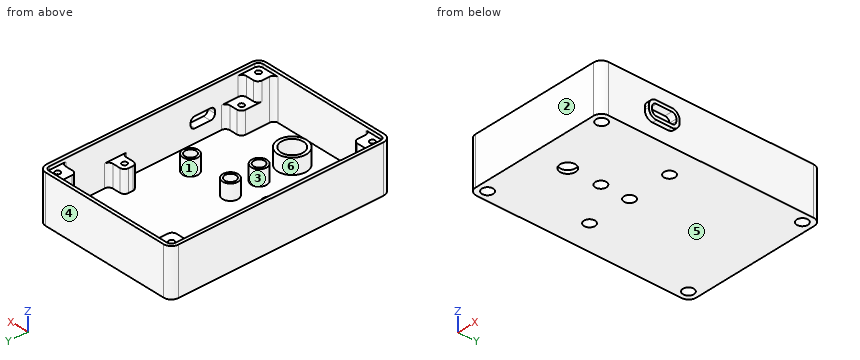
from build123d import *

# Parameters (mm, degrees)
SKETCH_1_W              = 66
SKETCH_1_H              = 100
SKETCH_1_W_2            = 63
SKETCH_1_H_2            = 97
EXTRUDE_1_DEPTH         = 20
SKETCH_3_W              = 66
SKETCH_3_H              = 100
EXTRUDE_2_DEPTH         = 1.5
SKETCH_4_W              = 7.5
SKETCH_4_H              = 6
SKETCH_4_H_2            = 7.5
EXTRUDE_3_DEPTH         = 10
HOLE_WIZARD_M2_21_D     = 2.3
HOLE_WIZARD_M2_21_DEPTH = 4
HOLE_WIZARD_M2_21_TIP   = 0.690989712
SKETCH_8_W              = 7.5
SKETCH_8_H              = 7.5
EXTRUDE_4_DEPTH         = 18.5
FILLET_1_R              = 2
FILLET_3_R              = 2
FILLET_4_R              = 3.5
SKETCH_9_R              = 2.5
SKETCH_9_R_2            = 3.5
CUT_EXTRUDE_1_DEPTH     = 64.158530699
EXTRUDE_START           = 7
SKETCH_10_R             = 3.5
SKETCH_10_R_2           = 2.5
EXTRUDE_5_DEPTH         = 7
SKETCH_11_R             = 2.5
CUT_EXTRUDE_2_DEPTH     = 18.5
HOLE_WIZARD_M21_D       = 2.4
SKETCH_15_W             = 5
SKETCH_15_H             = 11
CUT_EXTRUDE_3_DEPTH     = 85.025293811
FILLET_5_R              = 2
SKETCH_16_R             = 6.5
SKETCH_16_R_2           = 5
EXTRUDE_6_DEPTH         = 7
EXTRUDE_START_2         = 2
EXTRUDE_7_DEPTH         = 2


with BuildPart() as part:
    # Эскиз1 → Бобышка-Вытянуть1 (new body)
    with BuildSketch(Plane.XY):
        Rectangle(SKETCH_1_W, SKETCH_1_H)
        Rectangle(SKETCH_1_W_2, SKETCH_1_H_2, mode=Mode.SUBTRACT)
    extrude(amount=EXTRUDE_1_DEPTH)

    # Эскиз3 → Бобышка-Вытянуть2 (add)
    with BuildSketch(Plane(origin=(0, 0, 0), x_dir=(-1, 0, 0), z_dir=(0, 0, -1))):
        Rectangle(SKETCH_3_W, SKETCH_3_H)
    extrude(amount=EXTRUDE_2_DEPTH)

    # Эскиз4 → Бобышка-Вытянуть3 (add)
    with BuildSketch(Plane.XY):
        with Locations((-27.75, 16.5)):
            Rectangle(SKETCH_4_W, SKETCH_4_H)
        with Locations((27.75, 16.5)):
            Rectangle(SKETCH_4_W, SKETCH_4_H)
        with Locations((-27.75, -37.25)):
            Rectangle(SKETCH_4_W, SKETCH_4_H_2)
        with Locations((27.75, -37.25)):
            Rectangle(SKETCH_4_W, SKETCH_4_H_2)
    extrude(amount=EXTRUDE_3_DEPTH)

    # Сверло под метчик  спиральное M2.21
    with Locations(Plane.XY.offset(10)):
        with Locations((-27, 16.5), (27, 16.5), (27, -36.5), (-27, -36.5)):
            Hole(HOLE_WIZARD_M2_21_D / 2, depth=HOLE_WIZARD_M2_21_DEPTH)
            with Locations((0, 0, -(HOLE_WIZARD_M2_21_DEPTH + HOLE_WIZARD_M2_21_TIP / 2))):  # 118° drill point
                Cone(0, HOLE_WIZARD_M2_21_D / 2, HOLE_WIZARD_M2_21_TIP, mode=Mode.SUBTRACT)

    # Эскиз8 → Бобышка-Вытянуть4 (add)
    with BuildSketch(Plane.XY):
        with Locations((-27.75, 44.75)):
            Rectangle(SKETCH_8_W, SKETCH_8_H)
        with Locations((27.75, 44.75)):
            Rectangle(SKETCH_8_W, SKETCH_8_H)
        with Locations((27.75, -44.75)):
            Rectangle(SKETCH_8_W, SKETCH_8_H)
        with Locations((-27.75, -44.75)):
            Rectangle(SKETCH_8_W, SKETCH_8_H)
    extrude(amount=EXTRUDE_4_DEPTH)

    # Скругление1
    fillet_1_edges = [part.edges().sort_by_distance(p)[0] for p in [
        (-31.5, 41, 9.25),
        (-24, 41, 9.25),
        (-24, 48.5, 9.25),
        (31.5, 41, 9.25),
        (24, 48.5, 9.25),
        (24, 41, 9.25),
        (24, -48.5, 9.25),
        (-24, -48.5, 9.25),
        (-31.5, 19.5, 5),
        (-31.5, 13.5, 5),
        (-24, 13.5, 5),
        (-24, 19.5, 5),
        (31.5, 13.5, 5),
        (31.5, 19.5, 5),
        (24, 19.5, 5),
        (24, 13.5, 5),
        (-31.5, -33.5, 5),
        (-24, -33.5, 5),
        (31.5, -33.5, 5),
        (24, -33.5, 5),
    ]]
    fillet(fillet_1_edges, radius=FILLET_1_R)

    # Скругление3
    fillet_3_edges = [part.edges().sort_by_distance(p)[0] for p in [
        (31.5, -41, 14.25),
        (24, -41, 14.25),
        (-24, -41, 14.25),
        (31.5, -48.5, 19.25),
        (-31.5, -41, 14.25),
        (31.5, 48.5, 19.25),
        (-31.5, 48.5, 19.25),
        (-31.5, -48.5, 19.25),
    ]]
    fillet(fillet_3_edges, radius=FILLET_3_R)

    # Скругление4
    fillet_4_edges = [part.edges().sort_by_distance(p)[0] for p in [
        (33, -50, 9.25),
        (-33, -50, 9.25),
        (-33, 50, 9.25),
        (33, 50, 9.25),
    ]]
    fillet(fillet_4_edges, radius=FILLET_4_R)

    # Эскиз9 → Вырез-Вытянуть1 (cut, through all)
    with BuildSketch(Plane.XY):
        with Locations((-20, -7)):
            Circle(SKETCH_9_R)
        with Locations((20, -7)):
            Circle(SKETCH_9_R)
        with Locations((0, -20)):
            Circle(SKETCH_9_R)
        with Locations((0, -7)):
            Circle(SKETCH_9_R)
        with Locations((0, -35)):
            Circle(SKETCH_9_R_2)
    extrude(amount=-CUT_EXTRUDE_1_DEPTH, mode=Mode.SUBTRACT)

    # Эскиз10 → Бобышка-Вытянуть5 (add)
    # profile 1 of 4: a face of its own
    with BuildSketch(Plane.XY.offset(EXTRUDE_START)):
        with Locations(Location((0, -7, 0), (0, 0, 180))):
            Circle(SKETCH_10_R)
        with Locations((0, -7)):
            Circle(SKETCH_10_R_2, mode=Mode.SUBTRACT)
    # profile 2 of 4: a face of its own
    with BuildSketch(Plane.XY.offset(EXTRUDE_START)):
        with Locations(Location((20, -7, 0), (0, 0, 180))):
            Circle(SKETCH_10_R)
        with Locations((20, -7)):
            Circle(SKETCH_10_R_2, mode=Mode.SUBTRACT)
    # profile 3 of 4: a face of its own
    with BuildSketch(Plane.XY.offset(EXTRUDE_START)):
        with Locations(Location((0, -20, 0), (0, 0, 180))):
            Circle(SKETCH_10_R)
        with Locations((0, -20)):
            Circle(SKETCH_10_R_2, mode=Mode.SUBTRACT)
    # profile 4 of 4: a face of its own
    with BuildSketch(Plane.XY.offset(EXTRUDE_START)):
        with Locations(Location((-20, -7, 0), (0, 0, 180))):
            Circle(SKETCH_10_R)
        with Locations((-20, -7)):
            Circle(SKETCH_10_R_2, mode=Mode.SUBTRACT)
    extrude(amount=-EXTRUDE_5_DEPTH)

    # Эскиз11 → Вырез-Вытянуть2 (cut)
    with BuildSketch(Plane(origin=(0, 0, -1.5), x_dir=(-1, 0, 0), z_dir=(0, 0, -1))):
        with Locations((-28.5, 45.5)):
            Circle(SKETCH_11_R)
        with Locations((28.5, 45.5)):
            Circle(SKETCH_11_R)
        with Locations((28.5, -45.5)):
            Circle(SKETCH_11_R)
        with Locations((-28.5, -45.5)):
            Circle(SKETCH_11_R)
    extrude(amount=-CUT_EXTRUDE_2_DEPTH, mode=Mode.SUBTRACT)

    # Отверстие с зазором M21 (through all)
    with Locations(Plane(origin=(0, 0, 17), x_dir=(-1, 0, 0), z_dir=(0, 0, -1))):
        with Locations((-28.5, 45.5), (28.5, 45.5), (28.5, -45.5), (-28.5, -45.5)):
            Hole(HOLE_WIZARD_M21_D / 2)

    # Эскиз15 → Вырез-Вытянуть3 (cut, through all)
    with BuildSketch(Plane.ZY.offset(-31.5)):
        with Locations((8.5, -23)):
            Rectangle(SKETCH_15_W, SKETCH_15_H)
    extrude(amount=-CUT_EXTRUDE_3_DEPTH, mode=Mode.SUBTRACT)

    # Скругление5
    fillet_5_edges = [part.edges().sort_by_distance(p)[0] for p in [
        (32.25, -28.5, 6),
        (32.25, -17.5, 6),
        (32.25, -17.5, 11),
        (32.25, -28.5, 11),
    ]]
    fillet(fillet_5_edges, radius=FILLET_5_R)

    # Эскиз16 → Бобышка-Вытянуть6 (add)
    with BuildSketch(Plane.XY):
        with Locations(Location((0, -35, 0), (0, 0, 180))):
            Circle(SKETCH_16_R)
        with Locations((0, -35)):
            Circle(SKETCH_16_R_2, mode=Mode.SUBTRACT)
    extrude(amount=EXTRUDE_6_DEPTH)

    # Эскиз19 → Бобышка-Вытянуть7 (add)
    with BuildSketch(Plane(origin=(33, 0, 0), x_dir=(0, 0, -1), z_dir=(1, 0, 0)).offset(EXTRUDE_START_2)):
        with BuildLine():
            Line((-4.5, -26.5), (-4.5, -19.5))
            ThreePointArc((-4.5, -19.5), (-5.525126266, -17.025126266), (-8, -16))
            Line((-8, -16), (-9, -16))
            ThreePointArc((-9, -16), (-11.474873734, -17.025126266), (-12.5, -19.5))
            Line((-12.5, -19.5), (-12.5, -26.5))
            ThreePointArc((-12.5, -26.5), (-11.474873734, -28.974873734), (-9, -30))
            Line((-9, -30), (-8, -30))
            ThreePointArc((-8, -30), (-5.525126266, -28.974873734), (-4.5, -26.5))
        make_face()
        with BuildLine():
            Line((-11, -19.5), (-11, -26.5))
            ThreePointArc((-11, -26.5), (-10.414213562, -27.914213562), (-9, -28.5))
            Line((-9, -28.5), (-8, -28.5))
            ThreePointArc((-8, -28.5), (-6.585786438, -27.914213562), (-6, -26.5))
            Line((-6, -26.5), (-6, -19.5))
            ThreePointArc((-6, -19.5), (-6.585786438, -18.085786438), (-8, -17.5))
            Line((-8, -17.5), (-9, -17.5))
            ThreePointArc((-9, -17.5), (-10.414213562, -18.085786438), (-11, -19.5))
        make_face(mode=Mode.SUBTRACT)
    extrude(amount=-EXTRUDE_7_DEPTH)


solid = part.part
Can you work these out from the model? Positions are in its coordinate system, mm. Face numbers are marked on the shaded views. A direction names the side the tool comes from. Coordinates: 2 decimals unless noted, no trailing zeros. Loops run counter-clockwise (first coordinate to the right, second up) from the corner with the lowest first, then second, coordinate; pieces in that order, holes last. Notation, with made-up numbers: M -36.75,-39.5 L -14.75,-39.5 A17 ccw -14.75,-24.5 Z; hole C 11.25,13.25 d1. An arc over 180 degrees is marked long. Return JSON: item names as keys, results as strings. Group by question number.
Item 1: If I drill on L1, parallel to Y at x = -28.5, z = 17.9; L2, parallel to Y at x = 20, z = 5.25; L3, parallel to Y at x = 7, z = 1.25, over which ranges is the centre line in solid material (lowest first)? Write a range as from..to.
Item 2: Thinking about a two-plate mould opening in Y: for the marked faces 3, 4, 5 and 6, which applies, released by +Y, released by -Y, zero draft, split by the parting line, or undercut?
Item 3: I'm going to push flat-ended pins straight in: pin 1 Ø3.5 at (x, y) = (1.5, -19) entering from +Z; pin 2 Ø1.4 at (x, y) = (-27, 16.5) entering from +Z; pin 3 Ø2 at (x, y) = (16, -18.5) entering from +Z. Where does each tip first touch, or does it pass through?
Item 4: Imagine slicing it at A-A (y = 45.5). Please give me the cut outline in (x, z).
Item 5: Imagine slicing it at B-B (x = -20). Please give me the cut outline in (y, z), and give its area (4 significant figures).
Item 6: Imagine slicing it at D-D (y = -2). Please give me the cut outline in (x, z).
Item 7: On a 3-axis mill with a long thin cutter (end or side, diameter ignored), from which of +Z, -Z, +X, -X, +Y, -Y can I reach the whole of each face in a straight line? I mean the marked faces 1 and 2. Say none if no direction works.
Item 8: Imagine slicing it at C-C (z = 13.75). Give the number of separate pieces and of enclosed holes in the cut face, and give its area (3 significant figures).
Verdict:
{
 "1": {"L1": "y = -50..-46.7, -44.3..-41, 41..44.3, 46.7..50", "L2": "y = -50..-48.5, -10.5..-9.5, -4.5..-3.5, 48.5..50", "L3": "y = -50..-48.5, 48.5..50"},
 "2": {"face 3": "undercut", "face 4": "released by +Y", "face 5": "zero draft", "face 6": "undercut"},
 "3": {"pin 1": "stops at z = 7", "pin 2": "stops at z = 5.73", "pin 3": "stops at z = 0"},
 "4": {"outline": "M -33,-1.5 L -31,-1.5 L -31,17 L -29.7,17 L -29.7,18.5 L -31.5,18.5 L -31.5,20 L -33,20 Z; M -27.3,17 L -26,17 L -26,-1.5 L 26,-1.5 L 26,17 L 27.3,17 L 27.3,18.5 L 24,18.5 L 24,0 L -24,0 L -24,18.5 L -27.3,18.5 Z; M 29.7,17 L 31,17 L 31,-1.5 L 33,-1.5 L 33,20 L 31.5,20 L 31.5,18.5 L 29.7,18.5 Z"},
 "5": {"outline": "M -50,-1.5 L -9.5,-1.5 L -9.5,7 L -10.5,7 L -10.5,0 L -48.5,0 L -48.5,20 L -50,20 Z; M -4.5,-1.5 L 50,-1.5 L 50,20 L 48.5,20 L 48.5,0 L -3.5,0 L -3.5,7 L -4.5,7 Z", "area": "216.5 mm^2"},
 "6": {"outline": "M -33,-1.5 L 33,-1.5 L 33,20 L 31.5,20 L 31.5,0 L -31.5,0 L -31.5,20 L -33,20 Z"},
 "7": {"face 1": "+Z", "face 2": "+Z, -Z, +X, -X, -Y"},
 "8": {"separate pieces": "1", "enclosed holes": "5", "area": "628 mm^2"}
}
